For this review, use the dimensioned drawing (mm, ordinates from the lowest corner) and the shaded views. A direction names the side the tool comes from. Round coordinates to 2 decimals unless told otherwise and drop trailing zeros. Write each loop counter-clockwise with the first axis right and the second up, starting at its lowest first coordinate (ties: lowest second). Pieces come first, ordered by that corner, then holes. Notation, with made-up numbers: M -7.75,18 L 5.25,18 A24 ccw 5.25,49 Z; hole C -36.75,-21.5 d9. An arc over 180 degrees is marked long. One line per question, with ' | ' between items. Start each with the question number.
Item 1: Add section B-B, the plane y = 9. State the section outline as (x, z) points, and give its area (3 significant figures).
Item 2: For L1, parallel to X at y = 8.75, z = 21.75; L2, parallel to Y at x = 6.75, z = 21.5 (1 decimal); L3, parallel to X at y = 11, z = 9.25 (1 decimal), list the stretches that pass through material, from the lowest coordinate up.
Item 3: Draft analysis for pull direction Y (two halves, no side actions). For the marked faces 1, 2 and 3, state which applies: released by +Y, released by -Y, zero draft, split by the parting line, or undercut.
Item 4: Add section A-A, the plane x = 9. State the section outline as (y, z) points, and give its area (3 significant figures).
Item 5: Add section D-D, the plane x = 4.5. State the section outline as (y, z) points, and give its area (3 significant figures).
Item 6: Add section C-C, the plane z = 26.75. State the section outline as (x, y) points.
Item 7: Machinability: for the marked faces 4 and 5, which of the approach directions +Z, -Z, +X, -X, +Y, -Y give a long, thin tool a straight path to every point of the face, cutting with its end or side? Answer none if there is none.
Item 8: Insertion check: pin 1 Ø1 at (y, z) = (7.5, 15) entering from +X; pin 2 Ø1 at (x, z) = (3.5, 21) entering from -Y; pin 3 Ø3 at (y, z) = (5, 16.5) entering from -X. Each pin has a flat end and moves straight along its axis. Give the tip position at first contact, or say it passes through.
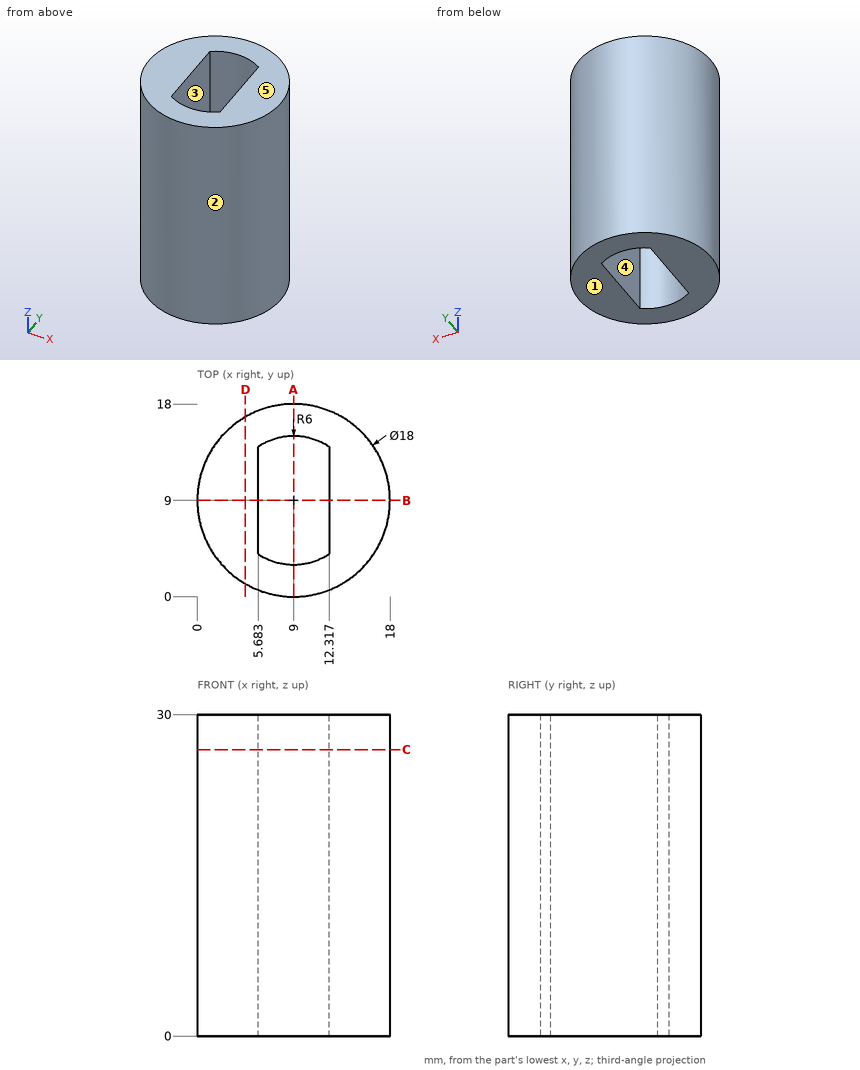
Computed values:
1) outline: M 0,0 L 5.68,0 L 5.68,30 L 0,30 Z; M 12.32,0 L 18,0 L 18,30 L 12.32,30 Z | area: 341 mm^2
2) L1: x = 0 to 5.68, 12.32 to 18 | L2: y = 0.3 to 3.4, 14.6 to 17.7 | L3: x = 0.2 to 5.7, 12.3 to 17.8
3) face 1: zero draft | face 2: split by the parting line | face 3: undercut
4) outline: M 0,0 L 3,0 L 3,30 L 0,30 Z; M 15,0 L 18,0 L 18,30 L 15,30 Z | area: 180 mm^2
5) outline: M 1.21,0 L 16.79,0 L 16.79,30 L 1.21,30 Z | area: 468 mm^2
6) outline: C 9,9 d18; hole M 5.68,4 A6 ccw 12.32,4 L 12.32,14 A6 ccw 5.68,14 Z
7) face 4: +Z, -Z | face 5: +Z, +X, -X, +Y, -Y
8) pin 1: stops at x = 17.94 | pin 2: stops at y = 1.52 | pin 3: stops at x = 0.35
